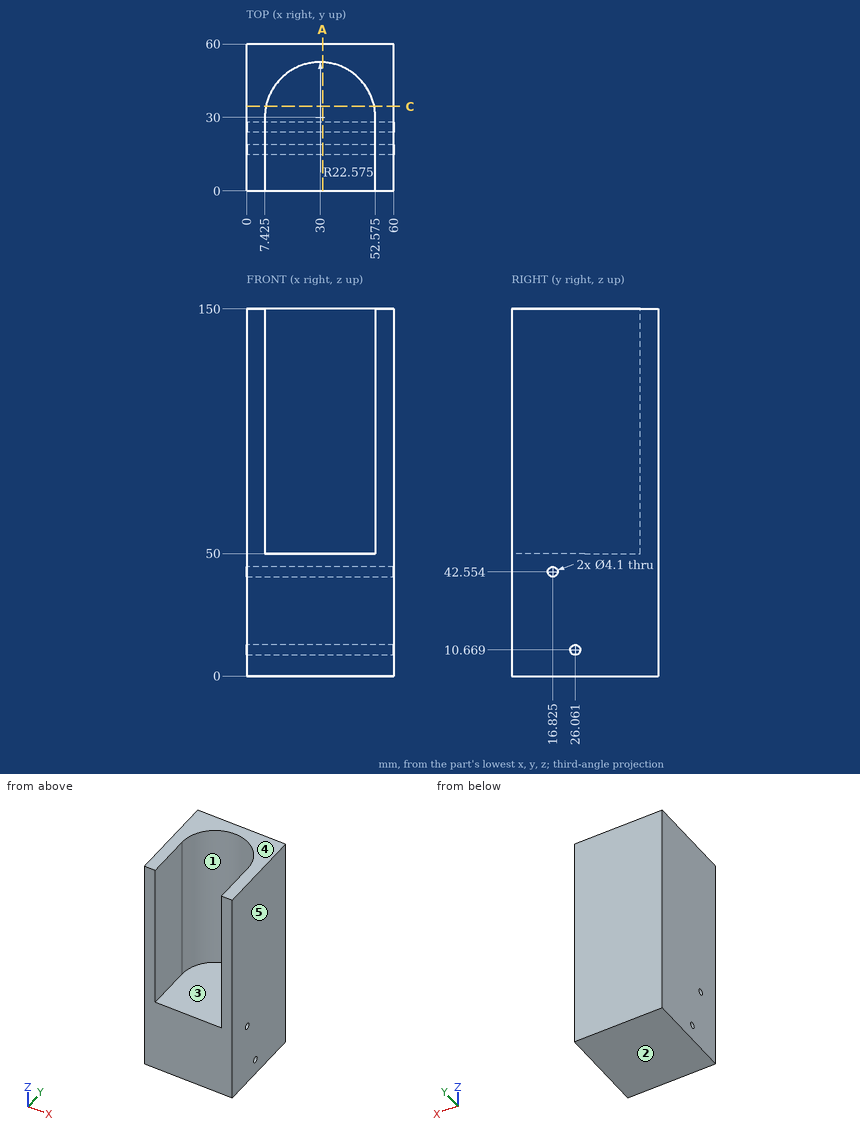
Drawing for the job (mm, zero at the part's lowest x, y, z). A direction names the side the tool comes from. Round coordinates to 2 decimals unless told otherwise and drop trailing zeros. Order: outer loops, then holes, each group sorted by start corner. A loop starts at its lowest first (then second) coordinate and runs counter-clockwise, first axis right, second up.
Item 1: Mould opens along X. For the marked faces 3, 4 and 5 say: pulls with the +X half, pulls with the -X half, needs draft (parallel to the pull), parting line crosses it, or undercut.
Item 2: Pin check, flat tips, straight feed: pin 1 (12 mm diameter, centred on x = 22, z = 90.5, fed in from -Y); pin 2 (22.5 mm diameter, centred on x = 21.5, y = 18.5, fed in from +Z); pin 3 (1.5 mm diameter, centred on x = 46.5, z = 106, fed in from -Y); pin 4 (2.5 mm diameter, centred on y = 16.83, z = 42.55, fed in from -X). Stop position of each tip, or through.
Item 3: Probe line 1 along X through (y, z) = (27.5, 53.5) (1 decimal); line 2 along Z through (x, y) = (30, 7); line 3 along X through (y, z) = (50, 72.5). List the from-to ranges inside material, lowest first.
Item 4: Saw through at C-C on y = 34.5. Write the cut outline in (x, z).
Item 5: Tool access for the marked faces 1 and 2: list every direction of +Z, -Z, +X, -X, +Y, -Y with a clear straight run to the whole face (end or side of a thin tool).
Item 6: Saw through at A-A on x = 31. State how many separate pieces and enclosed holes the cut face has, then the cut area to 3 significant figures.
Reported:
1. face 3: undercut
1. face 4: needs draft
1. face 5: pulls with the +X half
2. pin 1: stops at y = 47.71
2. pin 2: stops at z = 50
2. pin 3: stops at y = 44.56
2. pin 4: passes through
3. line 1: x = 0 to 7.4, 52.6 to 60
3. line 2: z = 0 to 50
3. line 3: x = 0 to 19.53, 40.47 to 60
4. outline: (0, 0) - (60, 0) - (60, 150) - (52.12, 150) - (52.12, 50) - (7.88, 50) - (7.88, 150) - (0, 150) - close
5. face 1: +Z, -Y
5. face 2: -Z, +X, -X, +Y, -Y
6. separate pieces: 1
6. enclosed holes: 2
6. area: 3,720 mm2
